Solid Edge part; units mm, degrees
sketch "Sketch1" plane through (0, 0, 0) normal (0, 0, 1) x (1, 0, 0)
  circle A0 centre (0, 0) radius 13.8
extrude "Ajout_matière_1" add sketch "Sketch1" along normal blind 35.5
sketch "Sketch2" plane through (0, 0, 0) normal (0, 0, 1) x (1, 0, 0)
  circle A0 centre (0, 0) radius 14.9
extrude "Ajout_matière_2" add sketch "Sketch2" along normal blind 24
sketch "Sketch3" plane through (0, 0, 0) normal (0, 0, -1) x (-1, 0, 0)
  circle A0 centre (0, 0) radius 4.85
extrude "Ajout_matière_3" add sketch "Sketch3" along normal blind 2
sketch "Sketch4" plane through (0, 0, -2) normal (0, 0, -1) x (-1, 0, 0)
  circle A0 centre (0, 0) radius 1
extrude "Ajout_matière_4" add sketch "Sketch4" along normal blind 7
hole "Perçage_1" at (8.5, 0, 0) direction (0, 0, 1) diameter 1.567 depth 30.8 thread major 2 thread length 2
hole "Hole1" at (-8.5, 0, 0) direction (0, 0, 1) diameter 1.567 depth 30.8 thread major 2 thread length 2
sketch "Sketch5" plane through (0, 0, 35.5) normal (0, 0, 1) x (0, 1, 0)
  circle A0 centre (0, 0) radius 5
extrude "Ajout_matière_5" add sketch "Sketch5" along normal blind 2.5
sketch "Sketch6" plane through (0, 0, 35.5) normal (0, 0, 1) x (-1, 0, 0)
  line L0 (-11.8, 2.5) -> (-9.8, 2.5)
  line L1 (-9.8, 2.5) -> (-9.8, -2.5)
  line L2 (-9.8, -2.5) -> (-11.8, -2.5)
  line L3 (-11.8, -2.5) -> (-11.8, 2.5)
  line L4 (9.8, 2.5) -> (11.8, 2.5)
  line L5 (11.8, 2.5) -> (11.8, -2.5)
  line L6 (11.8, -2.5) -> (9.8, -2.5)
  line L7 (9.8, -2.5) -> (9.8, 2.5)
  dimension "D1" = 11.8
  dimension "D2" = 9.8
  dimension "D3" = 11.8
  dimension "D4" = 9.8
extrude "Ajout_matière_7" add sketch "Sketch6" along normal blind 3
properties material "Acier S235"
Can you work these out from the model? Positions are in its coordinate system, mm. A direction names the side the tool comes from. Give positions to 0.01 mm unless a question says otherwise; leave off trailing zeros. Order: outer loops, then holes, each group sorted by start corner. A loop starts at its lowest first (then second) coordinate and runs counter-clockwise, first axis right, second up. Notation, with made-up numbers: M 15,8.5 L 23,8.5 A19 ccw 23,23.5 Z; hole C 68.5,-25.75 d4. An arc over 180 degrees is marked long. One line per item, written item: value.
Item 1: If we mould it in two halves opening along Y, with no side actions, what happens to faces 5 (the face through (-7.735, -0.17, 15.616)), 6 (the face through (-1.796, -13.683, 29.67)), 7 (the face through (10, -10, 24))? For each: pulls with the +Y half, pulls with the -Y half, needs draft (parallel to the pull), parting line crosses it, or undercut.
Verdict:
face 5: undercut
face 6: parting line crosses it
face 7: needs draft
Item 2: For faces 1 (the face through (-11.8, 0, 37)), 2 (the face through (8, 0, 30.8)), 3 (the face through (11, 2.5, 37)), 4 (the face through (9.8, 0, 37)), which set-ups out of +Z, -Z, +X, -X, +Y, -Y let a thin tool reach every point of the face, with its end or its side?
Verdict:
face 1: +Z, -X, +Y, -Y
face 2: -Z
face 3: +Z, +X, +Y
face 4: +Z, +Y, -Y
Item 3: If we section it at A-A on x = 0: Write out the boundary of the cut face in (y, z).
Verdict:
outline: M -14.9,0 L -4.85,0 L -4.85,-2 L -1,-2 L -1,-9 L 1,-9 L 1,-2 L 4.85,-2 L 4.85,0 L 14.9,0 L 14.9,24 L 13.8,24 L 13.8,35.5 L 5,35.5 L 5,38 L -5,38 L -5,35.5 L -13.8,35.5 L -13.8,24 L -14.9,24 Z
Item 4: If we section it at D-D on x = -11: Write out the boundary of the cut face in (y, z).
Verdict:
outline: M -10.05,0 L 10.05,0 L 10.05,24 L 8.33,24 L 8.33,35.5 L 2.5,35.5 L 2.5,38.5 L -2.5,38.5 L -2.5,35.5 L -8.33,35.5 L -8.33,24 L -10.05,24 Z
Item 5: For pin 1 (2.5 mm diameter, centred on y = 0, z = 36.5, fed in from -X); pin 2 (3 mm diameter, centred on x = -6, y = -4, fed in from +Z); pin 3 (1.6 mm diameter, centred on x = 11, z = 37.5, fed in from +Y), each with a flat end and sliding along its axis, tell me the tip position at first contact or that it passes through.
Verdict:
pin 1: x = -13.8
pin 2: z = 35.5
pin 3: y = 2.5
Item 6: If we section it at C-C on z = 34: Write out the boundary of the cut face in (x, y).
Verdict:
outline: C 0,0 d27.6
Item 7: If we section it at B-B on z = 6.5: Write out the boundary of the cut face in (x, y).
Verdict:
outline: C 0,0 d29.8; hole C -8.5,0 d1.57; hole C 8.5,0 d1.57
Item 8: Please list where these lines run through material, in increasing order: line 1 (Z direction, x = -3.75, y = 5.25); line 2 (Y direction, x = -8.5, z = 15.5); line 3 (Z direction, x = 1, y = 0.25).
Verdict:
line 1: 0 to 35.5
line 2: -12.24 to -0.78, 0.78 to 12.24
line 3: -2 to 38
